Verification items for this drawing (mm, ordinates from the low corner). Round coordinates to 2 decimals unless told otherwise and drop trailing zeros. Loops run counter-clockwise (first coordinate to the right, second up) from the corner with the lowest first, then second, coordinate; pieces in that order, holes last. Notation, with made-up numbers: (-37.75, 21) -> (-1.75, 21) arc R26 cw to (-1.75, 46) -> close; hole circle Ø7 at (37, 26.5). An arc over 180 degrees is marked (long way). One line per item, written item: value. Start each with the question number.
1. Cross-section at B-B on x = 7.5. Record the cut outline in (y, z), then the cut area to 3 significant figures.
2. Cross-section at D-D on y = 2.2. Record the cut outline in (x, z).
3. Release check for a two-part mould opening along Y. For the marked faces 1, 2, 3 and 4 record: +Y half, -Y half, draft (parallel to the pull), parting line (faces both ways), or undercut.
4. Cross-section at C-C on y = 0.7. Record the cut outline in (x, z).
5. Go/stop test with flat-tipped pins: pin 1 (1.5 mm diameter, centred on y = 1, z = 5, fed in from +X); pin 2 (1 mm diameter, centred on y = 1.5, z = 6.5, fed in from +X); pin 3 (1 mm diameter, centred on x = 12.5, y = 0.5, fed in from +Z). Record where each tip stops, or that it passes through.
6. Material ranges on L1, parallel to Z at x = 8.25, y = 2.3; L2, parallel to X at y = 0.75, z = 7.5; L3, parallel to Z at x = 7.5, y = 1.1, recorded low to high.
7. Cross-section at A-A on z = 7.5. Record the cut outline in (x, y).
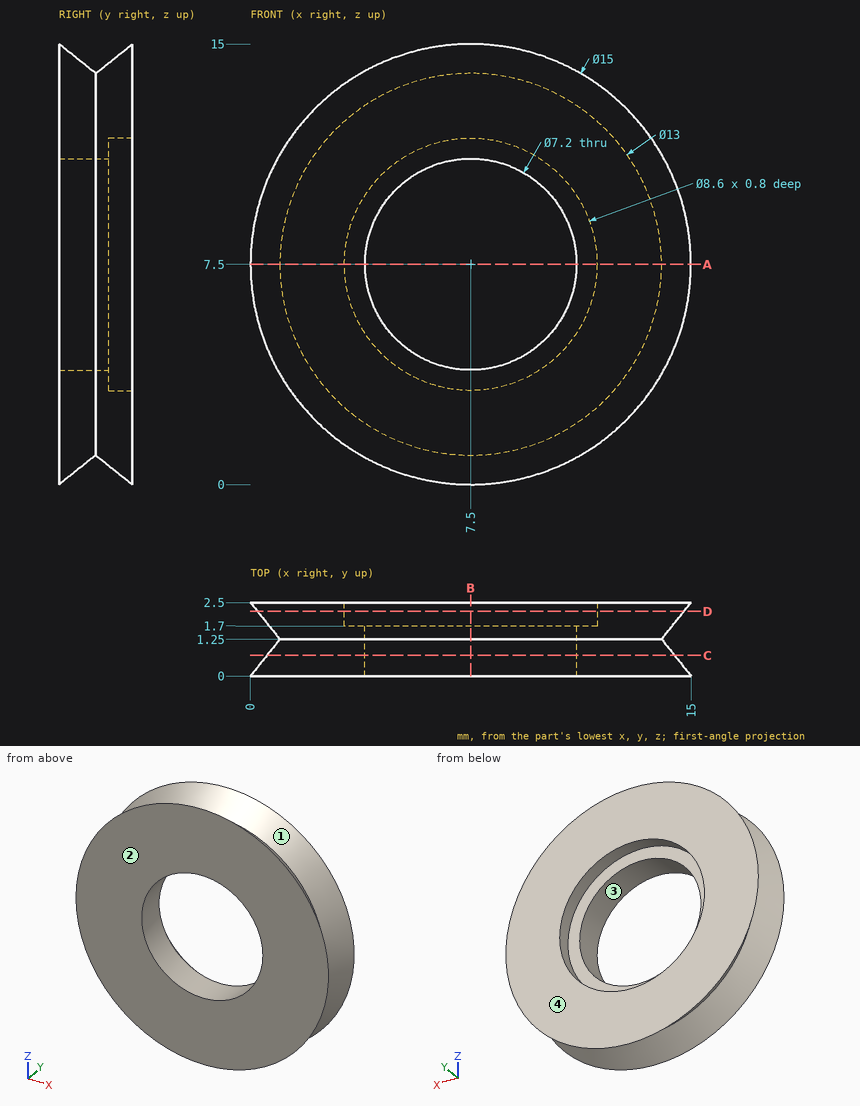
Taken from the geometry:
1. outline: (0, 0) -> (1.25, 1) -> (2.5, 0) -> (2.5, 3.2) -> (1.7, 3.2) -> (1.7, 3.9) -> (0, 3.9) -> close; (0, 11.1) -> (1.7, 11.1) -> (1.7, 11.8) -> (2.5, 11.8) -> (2.5, 15) -> (1.25, 14) -> (0, 15) -> close
1. area: 15.9 mm2
2. outline: circle Ø14.52 at (7.5, 7.5); hole circle Ø8.6 at (7.5, 7.5)
3. face 1: undercut
3. face 2: -Y half
3. face 3: draft
3. face 4: +Y half
4. outline: circle Ø13.88 at (7.5, 7.5); hole circle Ø7.2 at (7.5, 7.5)
5. pin 1: stops at x = 14.41
5. pin 2: stops at x = 14.53
5. pin 3: stops at z = 13.24
6. L1: z = 0.2 to 3.27, 11.73 to 14.8
6. L2: x = 0.6 to 3.9, 11.1 to 14.4
6. L3: z = 0.88 to 3.9, 11.1 to 14.12
7. outline: (0, 0) -> (3.9, 0) -> (3.9, 1.7) -> (3.2, 1.7) -> (3.2, 2.5) -> (0, 2.5) -> (1, 1.25) -> close; (11.1, 0) -> (15, 0) -> (14, 1.25) -> (15, 2.5) -> (11.8, 2.5) -> (11.8, 1.7) -> (11.1, 1.7) -> close
